```python
from build123d import *

# Parameters (mm, degrees)
MAIN_DEPTH               = 25
SKETCH2_R                = 20
PULLEY_HOLE_DEPTH        = 21
PULLEY_OUT_REACH         = 48
SKETCH3_W                = 10
SKETCH3_H                = 30
FIXATION_DEPTH           = 10
SKETCH5_R                = 3.5
BOSS_EXTRUDE3_DEPTH      = 4
M3_CLEARANCE_HOLE2_D     = 3.6
M3_CLEARANCE_HOLE2_DEPTH = 8
M3_CLEARANCE_HOLE3_D     = 3.6
M3_CLEARANCE_HOLE3_DEPTH = 10
M3_CLEARANCE_HOLE4_D     = 3.6
M3_CLEARANCE_HOLE4_DEPTH = 10
SKETCH15_R               = 3.25
CUT_EXTRUDE1_DEPTH       = 3.5


with BuildPart() as part:
    # Sketch1 → Main (new body)
    with BuildSketch(Plane.XY):
        with BuildLine():
            Line((-15.5, 23), (15.5, 23))
            ThreePointArc((15.5, 23), (20.803300859, 20.803300859), (23, 15.5))
            Line((23, 15.5), (23, -15.5))
            ThreePointArc((23, -15.5), (20.803300859, -20.803300859), (15.5, -23))
            Line((15.5, -23), (-15.5, -23))
            ThreePointArc((-15.5, -23), (-20.803300859, -20.803300859), (-23, -15.5))
            Line((-23, -15.5), (-23, 15.5))
            ThreePointArc((-23, 15.5), (-20.803300859, 20.803300859), (-15.5, 23))
        make_face()
    extrude(amount=MAIN_DEPTH)

    # Sketch2 → Pulley Hole (cut)
    with BuildSketch(Plane(origin=(0, 0, 0), x_dir=(-1, 0, 0), z_dir=(0, 0, -1))):
        Circle(SKETCH2_R)
    extrude(amount=-PULLEY_HOLE_DEPTH, mode=Mode.SUBTRACT)

    # Sketch3 → Pulley Out (cut, up to next)
    with BuildSketch(Plane.ZY.offset(23), mode=Mode.PRIVATE) as pulley_out_sk1:
        with Locations((13, 0)):
            Rectangle(SKETCH3_W, SKETCH3_H)
    pulley_out_tool1 = extrude(pulley_out_sk1.sketch, amount=-PULLEY_OUT_REACH, mode=Mode.PRIVATE) & part.part
    add(pulley_out_tool1.solids().sort_by_distance((-23, 0, 13))[0], mode=Mode.SUBTRACT)

    # Sketch4 → Fixation (add)
    with BuildSketch(Plane.XY.offset(25)):
        with BuildLine():
            Line((-7.5, -23), (7.5, -23))
            Line((7.5, -23), (7.5, -33))
            ThreePointArc((7.5, -33), (6.035533906, -36.535533906), (2.5, -38))
            Line((2.5, -38), (-2.5, -38))
            ThreePointArc((-2.5, -38), (-6.035533906, -36.535533906), (-7.5, -33))
            Line((-7.5, -33), (-7.5, -23))
        make_face()
        with BuildLine():
            Line((-7.5, 23), (7.5, 23))
            Line((7.5, 23), (7.5, 33))
            ThreePointArc((7.5, 33), (6.035533906, 36.535533906), (2.5, 38))
            Line((2.5, 38), (-2.5, 38))
            ThreePointArc((-2.5, 38), (-6.035533906, 36.535533906), (-7.5, 33))
            Line((-7.5, 33), (-7.5, 23))
        make_face()
    extrude(amount=-FIXATION_DEPTH)

    # Sketch5 → Boss-Extrude3 (add)
    with BuildSketch(Plane(origin=(0, 0, 21), x_dir=(-1, 0, 0), z_dir=(0, 0, -1))):
        Circle(SKETCH5_R)
    extrude(amount=BOSS_EXTRUDE3_DEPTH)

    # M3 Clearance Hole2
    with Locations(Plane.XY.offset(25)):
        with Locations((0, 0)):
            Hole(M3_CLEARANCE_HOLE2_D / 2, depth=M3_CLEARANCE_HOLE2_DEPTH)

    # M3 Clearance Hole3
    with Locations(Plane(origin=(0, -30.5, 25), x_dir=(1, 0, 0), z_dir=(0, 0, 1))):
        with Locations((0, 0)):
            Hole(M3_CLEARANCE_HOLE3_D / 2, depth=M3_CLEARANCE_HOLE3_DEPTH)

    # M3 Clearance Hole4
    with Locations(Plane(origin=(0, 30.5, 25), x_dir=(1, 0, 0), z_dir=(0, 0, 1))):
        with Locations((0, 0)):
            Hole(M3_CLEARANCE_HOLE4_D / 2, depth=M3_CLEARANCE_HOLE4_DEPTH)

    # Sketch15 → Cut-Extrude1 (cut)
    with BuildSketch(Plane.XY.offset(25)):
        Circle(SKETCH15_R)
    extrude(amount=-CUT_EXTRUDE1_DEPTH, mode=Mode.SUBTRACT)


solid = part.part
```
CAD build for the part. Positions are in the model's coordinates, mm. A direction names the side the tool comes from. Coordinates: 2 decimals unless noted, no trailing zeros. Order: outer loops, then holes, each group sorted by start corner. A loop starts at its lowest first (then second) coordinate and runs counter-clockwise, first axis right, second up.
(1) Pin check, flat tips, straight feed: pin 1 Ø7.5 at (x, y) = (1, 29) entering from -Z; pin 2 Ø5 at (x, z) = (-20.5, 12) entering from +Y; pin 3 Ø5 at (y, z) = (-29.5, 21) entering from -X; pin 4 Ø2 at (x, y) = (0, -30.5) entering from +Z. Stop position of each tip, or through.
Solution:
pin 1: stops at z = 15
pin 2: stops at y = 22.57
pin 3: stops at x = -7.5
pin 4: passes through
(2) Which spindle directions (+Z, -Z, +X, -X, +Y, -Y) get a long thin tool onto all of the face, cutting with end or side? Do faces 1 (the face through (2, 1, 17)), 2 (the face through (-3.233, -1.341, 19.028)), 3 (the face through (-18, -15, 13)). Say none if no direction does.
Solution:
face 1: -Z, -X
face 2: -Z
face 3: -X
(3) Drill centre lines: L1, parallel to Y at x = 0, z = 21.25; L2, parallel to Y at x = 0, z = 18.75; L3, parallel to Y at x = 0, z = 23.9. Where is each one in solid material? Low to high.
Solution:
L1: y = -38 to -32.3, -28.7 to -1.8, 1.8 to 28.7, 32.3 to 38
L2: y = -38 to -32.3, -28.7 to -20, -3.5 to -1.8, 1.8 to 3.5, 20 to 28.7, 32.3 to 38
L3: y = -38 to -32.3, -28.7 to -3.25, 3.25 to 28.7, 32.3 to 38
(4) Saw through at A-A, the plane y = 30.5. Write the cut outline in (x, z).
Solution:
outline: (-7.5, 15) - (-1.8, 15) - (-1.8, 25) - (-7.5, 25) - close; (1.8, 15) - (7.5, 15) - (7.5, 25) - (1.8, 25) - close
(5) Saw through at D-D, the plane y = 0. Write the cut outline in (x, z).
Solution:
outline: (-23, 0) - (-20, 0) - (-20, 8) - (-23, 8) - close; (-23, 18) - (-20, 18) - (-20, 21) - (-3.5, 21) - (-3.5, 17) - (-1.8, 17) - (-1.8, 21.5) - (-3.25, 21.5) - (-3.25, 25) - (-23, 25) - close; (1.8, 17) - (3.5, 17) - (3.5, 21) - (20, 21) - (20, 0) - (23, 0) - (23, 25) - (3.25, 25) - (3.25, 21.5) - (1.8, 21.5) - close
(6) Saw through at B-B, the plane z = 3.75. Write the cut outline in (x, y).
Solution:
outline: (-23, -15.5) arc R7.5 ccw to (-15.5, -23) - (15.5, -23) arc R7.5 ccw to (23, -15.5) - (23, 15.5) arc R7.5 ccw to (15.5, 23) - (-15.5, 23) arc R7.5 ccw to (-23, 15.5) - close; hole circle Ø40 at (0, 0)
(7) Saw through at C-C, the plane x = 0. Count the separate pieces of the cut face and the enclosed holes in it, and give its area (3 significant figures).
Solution:
separate pieces: 4
enclosed holes: 0
area: 527 mm2
(8) Mould opens along Y. For faces 4 (the face through (-20.4, -0.2, 8)), 5 (the face through (0, -38, 20)), 6 (the face through (20.745, 20.861, 12.325)), 7 (the face through (7.5, 28, 20)) say: released by +Y, released by -Y, zero draft, split by the parting line, or undercut.
Solution:
face 4: undercut
face 5: released by -Y
face 6: released by +Y
face 7: zero draft
